Answer from the drawing. Dimensions are ordinates in mm from the lowest x, y and z of the part. A direction names the side the tool comes from. Round coordinates to 2 decimals unless told otherwise and drop trailing zeros. Loops run counter-clockwise (first coordinate to the right, second up) from the corner with the lowest first, then second, coordinate; pieces in that order, holes last. Notation, with made-up numbers: M 42.5,28.5 L 58.5,28.5 A8 cw 58.5,38.5 Z; hole C 80,53.5 d11. An arc over 180 degrees is marked long. One line per item, written item: value.
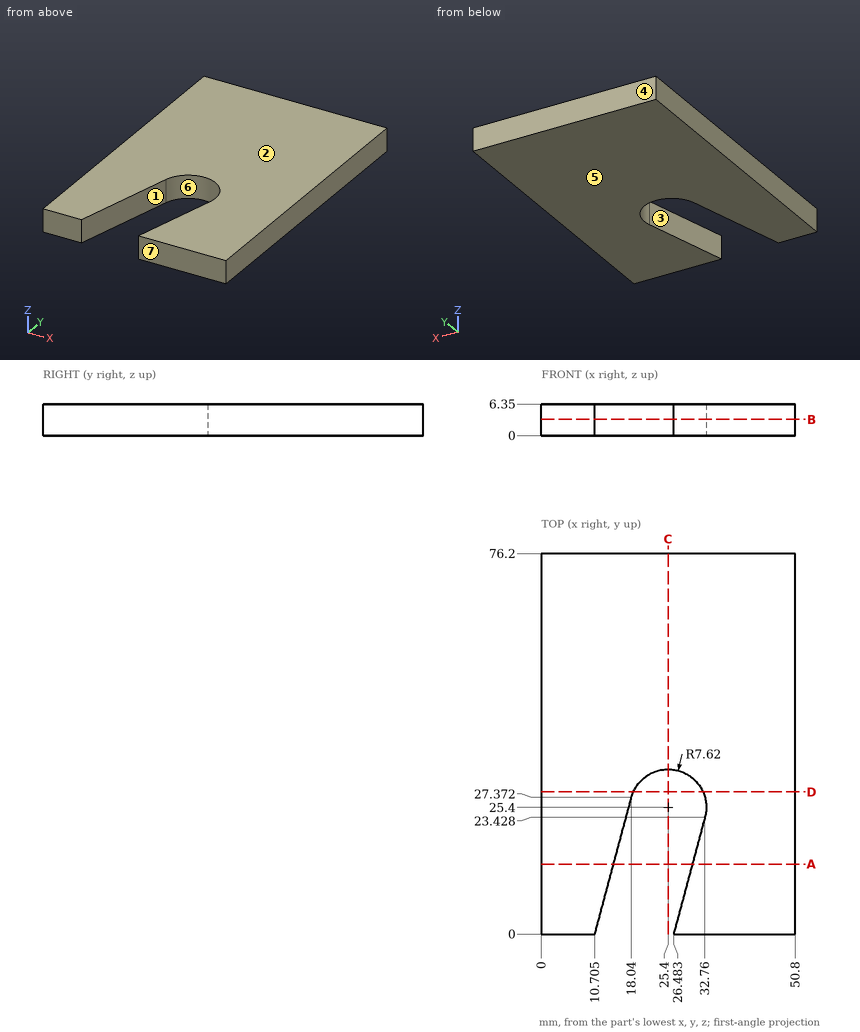
1) The mould has two halves that part along Y. Classify the marked faces 4, 5, 6 and 7: +Y half, -Y half, draft (parallel to the pull), parting line (faces both ways), or undercut.
Check values:
face 4: +Y half
face 5: draft
face 6: undercut
face 7: -Y half
2) Find the intervals of material crossed by probe 1 along X at (y, z) = (5, 6) (1 decimal); probe 2 along Y at (x, z) = (23.5, 3); probe 3 along Y at (x, z) = (25, 1), in increasing order. Write a range as from..to.
Check values:
probe 1: 0..12, 27.8..50.8
probe 2: 32.78..76.2
probe 3: 33.01..76.2
3) For the marked faces 1, 2 and 3, determine the directions among +Z, -Z, +X, -X, +Y, -Y from which every point of the face is accessible in a straight line to the end or side of a thin tool.
Check values:
face 1: +Z, -Z, -Y
face 2: +Z, +X, -X, +Y, -Y
face 3: +Z, -Z
4) Find section A-A (y = 14). Give the vertices of the cut face in (x, z), then the cut area to 3 significant figures.
Check values:
outline: M 0,0 L 14.46,0 L 14.46,6.35 L 0,6.35 Z; M 30.23,0 L 50.8,0 L 50.8,6.35 L 30.23,6.35 Z
area: 222 mm2
5) Find section D-D (y = 28.5). Give the vertices of the cut face in (x, z), then the cut area to 3 significant figures.
Check values:
outline: M 0,0 L 18.44,0 L 18.44,6.35 L 0,6.35 Z; M 32.36,0 L 50.8,0 L 50.8,6.35 L 32.36,6.35 Z
area: 234 mm2
6) Find section B-B (z = 3.25). Give the vertices of the cut face in (x, y) (1 decimal).
Check values:
outline: M 0,0 L 10.7,0 L 18,27.4 A7.6 cw 32.8,23.4 L 26.5,0 L 50.8,0 L 50.8,76.2 L 0,76.2 Z
7) Find section C-C (x = 25.4). Give the vertices of the cut face in (y, z), then the cut area to 3 significant figures.
Check values:
outline: M 33.02,0 L 76.2,0 L 76.2,6.35 L 33.02,6.35 Z
area: 274 mm2
8) This flat-tipped pin is pushed along its axis until it touches: pin 1 (1.5 mm diameter, centred on x = 24, z = 4.5, fed in from -Y). Where does it stop, or does it pass through?
Check values:
pin 1: y = 32.71
